Input: part model. Units: mm. Frame: model coordinates. Give positions to 0.01 mm unless a question says otherwise; leave off trailing zeros. Order: outer loops, then holes, each group sorted by start corner. A loop starts at its lowest first (then second) coordinate and runs counter-clockwise, first axis right, second up. Notation, with made-up numbers: (80, -25) - (114, -25) arc R19 ccw to (114, 3) - close; hole circle Ø2 at (-5.75, -10). An arc over 180 degrees is marked (long way). Answer in a Markdown table with one row per item. Add a question column.
1. Section query D-D on y = 1.5. Count the separate pieces of the cut face and the enclosed holes in it, and give its area (3 significant figures).
2. Ray query, line 1 (X direction, y = 0.15, z = -1035.5); line 2 (X direction, y = 2.4, z = -1054); line 3 (X direction, y = 1.45, z = -1059.5). Return the intervals inside material, ascending. Write a range as [from, to].
3. Section query A-A on z = -1037. Return loops of the section in (x, y).
4. Section query C-C on z = -1027.5. Return loops of the section in (x, y).
5. Contact query for flat-ended pins moving along their axis: pin 1 (1.3 mm diameter, centred on y = 1, z = -1020.5, fed in from +X); pin 2 (0.8 mm diameter, centred on x = 367, y = 1.5, fed in from +Z); pin 3 (0.8 mm diameter, centred on x = 365.24, z = -1033.86, fed in from +Y). Output: stop coordinate, or through.
6. Section query B-B on x = 332. Return loops of the section in (y, z), and give its area (3 significant figures).
```python
from build123d import *

# Parameters (mm, degrees)
SKETCH1_R           = 1.6
SKETCH1_R_2         = 1.75
SKETCH1_R_3         = 3.95
SKETCH1_R_4         = 12
BOSS_EXTRUDE1_DEPTH = 3


with BuildPart() as part:
    # Sketch1 → Boss-Extrude1 (new body)
    with BuildSketch(Plane(origin=(0, 0, 0), x_dir=(1, 0, 0), z_dir=(0, 1, 0))):
        with BuildLine():
            Line((312.373352996, 1022.190294437), (327.907309833, 1022.190294437))
            ThreePointArc((327.907309833, 1022.190294437), (328.157309833, 1022.257281735), (328.340322535, 1022.440294437))
            ThreePointArc((328.340322535, 1022.440294437), (329.126888323, 1022.543848684), (329.023336329, 1021.757282599))
            ThreePointArc((329.023336329, 1021.757282599), (328.840324865, 1021.574270305), (328.773337833, 1021.324271437))
            Line((328.773337833, 1021.324271437), (328.773337833, 1019.690242437))
            ThreePointArc((328.773337833, 1019.690242437), (328.919784442, 1019.336689047), (329.273337833, 1019.190242437))
            Line((329.273337833, 1019.190242437), (334.273335833, 1019.190242437))
            ThreePointArc((334.273335833, 1019.190242437), (334.626889492, 1019.336688397), (334.773336751, 1019.690241519))
            Line((334.773336751, 1019.690241519), (334.773336751, 1021.324268519))
            ThreePointArc((334.773336751, 1021.324268519), (334.706349307, 1021.57426848), (334.523336498, 1021.757281075))
            ThreePointArc((334.523336498, 1021.757281075), (334.419781792, 1022.543846802), (335.206347937, 1022.440295269))
            ThreePointArc((335.206347937, 1022.440295269), (335.389360338, 1022.257283911), (335.639359245, 1022.190297025))
            Line((335.639359245, 1022.190297025), (340.773337745, 1022.190297025))
            Line((340.773337745, 1022.190297025), (340.773337745, 1024.990297025))
            Line((340.773337745, 1024.990297025), (339.423337745, 1024.990297025))
            Line((339.423337745, 1024.990297025), (339.423337745, 1029.190297025))
            Line((339.423337745, 1029.190297025), (340.773337745, 1029.190297025))
            Line((340.773337745, 1029.190297025), (340.773337745, 1032.190297025))
            Line((340.773337745, 1032.190297025), (343.973337745, 1032.190297025))
            Line((343.973337745, 1032.190297025), (343.973337745, 1029.190297025))
            Line((343.973337745, 1029.190297025), (345.323337745, 1029.190297025))
            Line((345.323337745, 1029.190297025), (345.323337745, 1024.990292188))
            Line((345.323337745, 1024.990292188), (343.973337745, 1024.990292188))
            Line((343.973337745, 1024.990292188), (343.973337745, 1022.190292188))
            Line((343.973337745, 1022.190292188), (349.107314245, 1022.190292188))
            ThreePointArc((349.107314245, 1022.190292188), (349.357314245, 1022.257279486), (349.540326947, 1022.440292188))
            ThreePointArc((349.540326947, 1022.440292188), (350.326891976, 1022.543845827), (350.223341741, 1021.75728035))
            ThreePointArc((350.223341741, 1021.75728035), (350.040330277, 1021.574268055), (349.973343245, 1021.324269188))
            Line((349.973343245, 1021.324269188), (349.973343245, 1019.690240188))
            ThreePointArc((349.973343245, 1019.690240188), (350.119789854, 1019.336686797), (350.473343245, 1019.190240188))
            Line((350.473343245, 1019.190240188), (355.473340245, 1019.190240188))
            ThreePointArc((355.473340245, 1019.190240188), (355.826893904, 1019.336686148), (355.973341163, 1019.69023927))
            Line((355.973341163, 1019.69023927), (355.973341163, 1021.32426627))
            ThreePointArc((355.973341163, 1021.32426627), (355.906353816, 1021.574266257), (355.723341079, 1021.757278924))
            ThreePointArc((355.723341079, 1021.757278924), (355.619786681, 1022.543844692), (356.406352785, 1022.44029285))
            ThreePointArc((356.406352785, 1022.44029285), (356.589365548, 1022.257281171), (356.839364996, 1022.190294437))
            Line((356.839364996, 1022.190294437), (372.373340046, 1022.190294437))
            Line((372.373340046, 1022.190294437), (372.373340046, 1072.190301225))
            ThreePointArc((372.373340046, 1072.190301225), (370.908875012, 1075.72583207), (367.373345046, 1077.190299225))
            Line((367.373345046, 1077.190299225), (317.373348046, 1077.190299225))
            ThreePointArc((317.373348046, 1077.190299225), (313.837816014, 1075.725834155), (312.373352996, 1072.190301275))
            Line((312.373352996, 1072.190301275), (312.373352996, 1022.190294437))
        make_face()
        with Locations((366.893344996, 1047.842461747)):
            Circle(SKETCH1_R, mode=Mode.SUBTRACT)
        with Locations((357.873345496, 1071.990299275)):
            Circle(SKETCH1_R_2, mode=Mode.SUBTRACT)
        with Locations((357.873345496, 1040.990299275)):
            Circle(SKETCH1_R_2, mode=Mode.SUBTRACT)
        with Locations((322.373345996, 1056.490299275)):
            Circle(SKETCH1_R_3, mode=Mode.SUBTRACT)
        with Locations((342.373345496, 1056.490299275)):
            Circle(SKETCH1_R_4, mode=Mode.SUBTRACT)
        with Locations((326.873345496, 1071.990299275)):
            Circle(SKETCH1_R_2, mode=Mode.SUBTRACT)
        with Locations((326.873345496, 1040.990299275)):
            Circle(SKETCH1_R_2, mode=Mode.SUBTRACT)
        with Locations((317.853347996, 1047.84952041)):
            Circle(SKETCH1_R, mode=Mode.SUBTRACT)
        with BuildLine():
            Line((365.243389653, 1060.95296097), (365.243389653, 1056.48501097))
            ThreePointArc((365.243389653, 1056.48501097), (365.176400533, 1056.235010504), (364.993385671, 1056.051998658))
            ThreePointArc((364.993385671, 1056.051998658), (364.889836092, 1055.26543287), (365.676401176, 1055.368987799))
            ThreePointArc((365.676401176, 1055.368987799), (365.859413353, 1055.55200075), (366.109412996, 1055.618988627))
            Line((366.109412996, 1055.618988627), (367.677282996, 1055.618988627))
            ThreePointArc((367.677282996, 1055.618988627), (367.927282247, 1055.552001761), (368.110294834, 1055.368990124))
            ThreePointArc((368.110294834, 1055.368990124), (368.896860423, 1055.26543905), (368.793306996, 1056.052004329))
            ThreePointArc((368.793306996, 1056.052004329), (368.610294145, 1056.235017289), (368.543306996, 1056.485017627))
            Line((368.543306996, 1056.485017627), (368.543306996, 1060.952967627))
            ThreePointArc((368.543306996, 1060.952967627), (368.610293862, 1061.202966879), (368.793305499, 1061.385979465))
            ThreePointArc((368.793305499, 1061.385979465), (368.89685718, 1062.172545813), (368.110291294, 1062.068990627))
            ThreePointArc((368.110291294, 1062.068990627), (367.927278767, 1061.885978026), (367.677278996, 1061.818990627))
            Line((367.677278996, 1061.818990627), (366.109410996, 1061.818990627))
            ThreePointArc((366.109410996, 1061.818990627), (365.859411616, 1061.885977015), (365.676398679, 1062.068988302))
            ThreePointArc((365.676398679, 1062.068988302), (364.889832133, 1062.172538478), (364.993388824, 1061.38597279))
            ThreePointArc((364.993388824, 1061.38597279), (365.176401775, 1061.202960613), (365.243389653, 1060.95296097))
        make_face(mode=Mode.SUBTRACT)
        with BuildLine():
            Line((316.203388653, 1039.193570463), (316.203388653, 1034.725621463))
            ThreePointArc((316.203388653, 1034.725621463), (316.136399531, 1034.475620993), (315.953384663, 1034.292609147))
            ThreePointArc((315.953384663, 1034.292609147), (315.849835095, 1033.506043359), (316.636400176, 1033.609598291))
            ThreePointArc((316.636400176, 1033.609598291), (316.819412786, 1033.792611493), (317.069412996, 1033.85959912))
            Line((317.069412996, 1033.85959912), (318.637282996, 1033.85959912))
            ThreePointArc((318.637282996, 1033.85959912), (318.887282247, 1033.792612254), (319.070294834, 1033.609600616))
            ThreePointArc((319.070294834, 1033.609600616), (319.856860423, 1033.506049543), (319.753306996, 1034.292614822))
            ThreePointArc((319.753306996, 1034.292614822), (319.570294395, 1034.475627349), (319.503306996, 1034.72562712))
            Line((319.503306996, 1034.72562712), (319.503306996, 1039.19357712))
            ThreePointArc((319.503306996, 1039.19357712), (319.570293862, 1039.443576372), (319.753305499, 1039.626588958))
            ThreePointArc((319.753305499, 1039.626588958), (319.856856573, 1040.413154547), (319.070291294, 1040.30960112))
            ThreePointArc((319.070291294, 1040.30960112), (318.887278334, 1040.126588269), (318.637277996, 1040.05960112))
            Line((318.637277996, 1040.05960112), (317.069410996, 1040.05960112))
            ThreePointArc((317.069410996, 1040.05960112), (316.819411616, 1040.126587508), (316.636398679, 1040.309598795))
            ThreePointArc((316.636398679, 1040.309598795), (315.849832892, 1040.413148364), (315.953387824, 1039.626583283))
            ThreePointArc((315.953387824, 1039.626583283), (316.136401025, 1039.443570673), (316.203388653, 1039.193570463))
        make_face(mode=Mode.SUBTRACT)
        with BuildLine():
            Line((368.543303996, 1034.72562712), (368.543303996, 1039.19357712))
            ThreePointArc((368.543303996, 1039.19357712), (368.610290862, 1039.443576372), (368.793302499, 1039.626588958))
            ThreePointArc((368.793302499, 1039.626588958), (368.896853573, 1040.413154547), (368.110288294, 1040.30960112))
            ThreePointArc((368.110288294, 1040.30960112), (367.927275767, 1040.126588519), (367.677275996, 1040.05960112))
            Line((367.677275996, 1040.05960112), (366.109407996, 1040.05960112))
            ThreePointArc((366.109407996, 1040.05960112), (365.859408616, 1040.126587508), (365.676395679, 1040.309598795))
            ThreePointArc((365.676395679, 1040.309598795), (364.889829133, 1040.413148971), (364.993385824, 1039.626583283))
            ThreePointArc((364.993385824, 1039.626583283), (365.176399025, 1039.443570673), (365.243386653, 1039.193570463))
            Line((365.243386653, 1039.193570463), (365.243386653, 1034.725621463))
            ThreePointArc((365.243386653, 1034.725621463), (365.176397531, 1034.475620993), (364.993382663, 1034.292609147))
            ThreePointArc((364.993382663, 1034.292609147), (364.889833095, 1033.506043359), (365.676398176, 1033.609598291))
            ThreePointArc((365.676398176, 1033.609598291), (365.859410353, 1033.792611243), (366.109409996, 1033.85959912))
            Line((366.109409996, 1033.85959912), (367.677279996, 1033.85959912))
            ThreePointArc((367.677279996, 1033.85959912), (367.927279247, 1033.792612254), (368.110291834, 1033.609600616))
            ThreePointArc((368.110291834, 1033.609600616), (368.896857423, 1033.506049543), (368.793303996, 1034.292614822))
            ThreePointArc((368.793303996, 1034.292614822), (368.610291395, 1034.475627349), (368.543303996, 1034.72562712))
        make_face(mode=Mode.SUBTRACT)
    extrude(amount=BOSS_EXTRUDE1_DEPTH)


solid = part.part
```
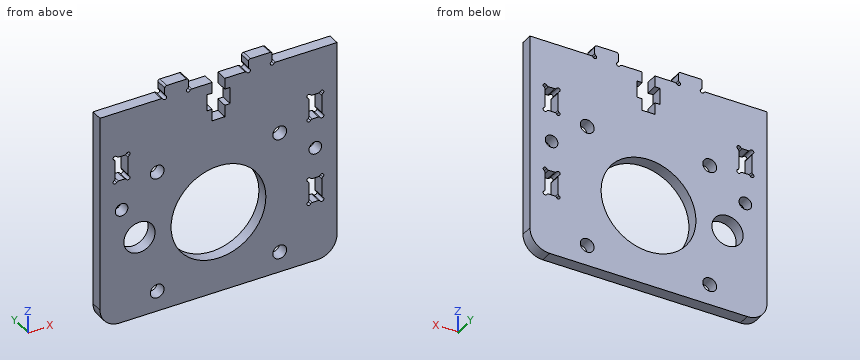
Answer:
| question | item | result |
|---|---|---|
| 1 | separate pieces | 1 |
| 1 | enclosed holes | 11 |
| 1 | area | 2,650 mm² |
| 2 | line 1 | x = [312.37, 316.2], [319.5, 365.24], [368.54, 372.37] |
| 2 | line 2 | x = [312.37, 319.31], [325.44, 330.63], [354.11, 372.37] |
| 2 | line 3 | x = [312.37, 319.82], [324.93, 330.76], [353.99, 365.24], [368.54, 372.37] |
| 3 | outline | (312.37, 0) - (316.2, 0) - (316.2, 3) - (312.37, 3) - close; (319.5, 0) - (365.24, 0) - (365.24, 3) - (319.5, 3) - close; (368.54, 0) - (372.37, 0) - (372.37, 3) - (368.54, 3) - close |
| 4 | outline | (312.37, 0) - (339.42, 0) - (339.42, 3) - (312.37, 3) - close; (345.32, 0) - (372.37, 0) - (372.37, 3) - (345.32, 3) - close |
| 5 | pin 1 | stops at x = 355.97 |
| 5 | pin 2 | stops at z = -1022.19 |
| 5 | pin 3 | passes through |
| 6 | outline | (0, -1077.19) - (3, -1077.19) - (3, -1062.52) - (0, -1062.52) - close; (0, -1050.46) - (3, -1050.46) - (3, -1019.19) - (0, -1019.19) - close |
| 6 | area | 138 mm² |
